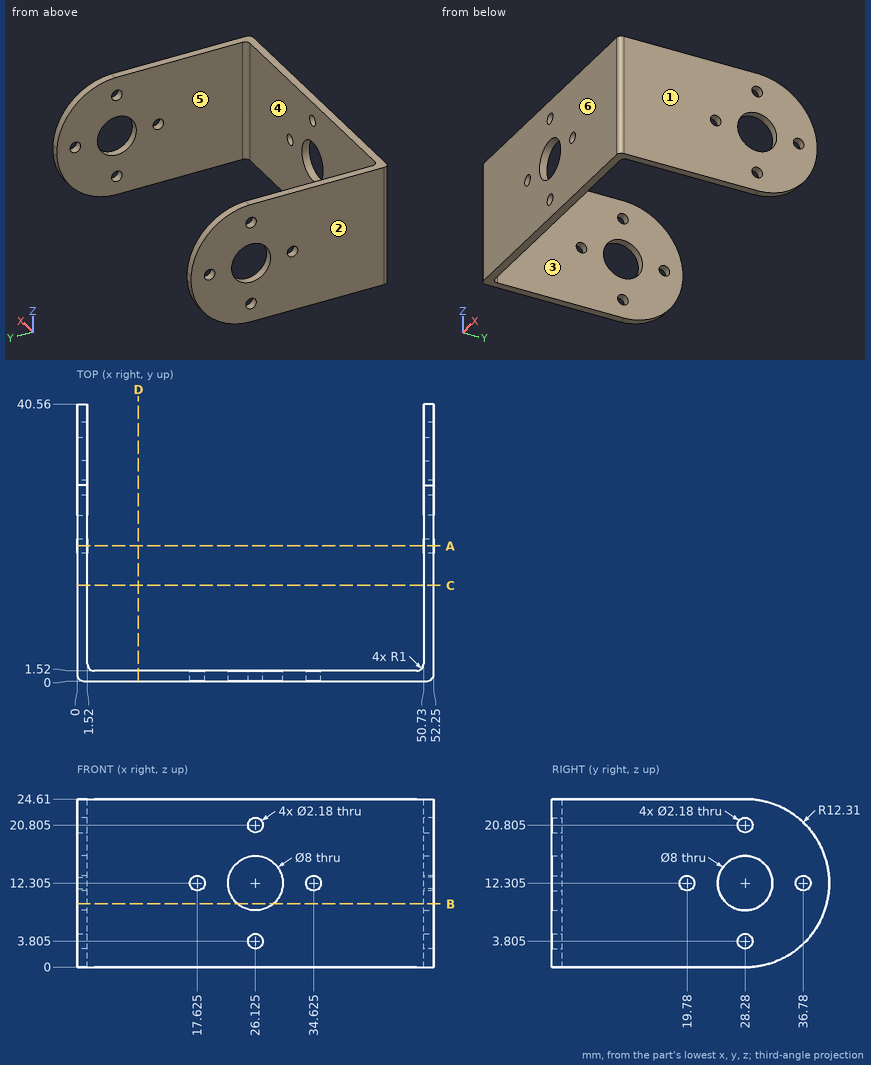
Geometry: see drawing. Coordinates: mm, zero at the bounding-box minimum. A direction names the side the tool comes from. Coordinates: 2 decimals unless noted, no trailing zeros. Write each loop counter-clockwise with the first axis right and the second up, starting at its lowest first coordinate (ties: lowest second). Pieces come first, ordered by that corner, then holes. Notation, with made-up numbers: M -32.75,53.5 L -1.75,53.5 A9 cw -1.75,64.5 Z; hole C 48.5,11 d8. An arc over 180 degrees is marked long. Use CSV: the item, a comma, the result in double quotes. Start each with the question number.
1. Mould query, pull axis X, two halves, no side actions, for the marked faces 1, 2, 3 and 4. Classes: pulls with the +X half, pulls with the -X half, needs draft (parallel to the pull), parting line crosses it, or undercut.
2. Cut plane A-A on y = 19.78. Return the cut outline in (x, z) (3 decimals), plus the area to 3 significant figures.
3. First-contact query: P1, Ø4, axis at x = 39, z = 6.5, coming from the +Y side; P2, Ø1.7, axis at y = 28.28, z = 3.805, coming from the +X side; P3, Ø12, axis at x = 46, y = 34.5, coming from the -Z side. Flat tips, straight axial feed; report the tip coordinate or a pass-through.
4. Cut plane D-D on x = 9. Return the cut outline in (y, z).
5. Cut plane B-B on z = 9.25. Return the cut outline in (x, y), plus the area to 3 significant figures.
6. Reachability of the marked faces 5 and 6 from +Z, -Z, +X, -X, +Y, -Y: full face, straight path, thin tool, end or side. Return the list, or none.
7. Ray query, probe 1 along X at (y, z) = (35.5, 14); probe 2 along Y at (x, z) = (37, 4.75); probe 3 along Z at (x, y) = (51.45, 19.78) (3 decimals). Return the intervals inside material, ascending.
8. Cut plane C-C on y = 14. Return the cut outline in (x, z).
Entries:
1,face 1,"pulls with the +X half"
1,face 2,"pulls with the -X half"
1,face 3,"undercut"
1,face 4,"undercut"
2,outline,"M 0,0 L 1.52,0 L 1.52,11.215 L 0,11.215 Z; M 0,13.395 L 1.52,13.395 L 1.52,24.61 L 0,24.61 Z; M 50.73,0 L 52.25,0 L 52.25,11.215 L 50.73,11.215 Z; M 50.73,13.395 L 52.25,13.395 L 52.25,24.61 L 50.73,24.61 Z"
2,area,"68.2 mm²"
3,P1,"y = 1.52"
3,P2,"through"
3,P3,"z = 0.26"
4,outline,"M 0,0 L 1.52,0 L 1.52,24.61 L 0,24.61 Z"
5,outline,"M 0,1 A1 ccw 1,0 L 23.54,0 L 23.54,1.52 L 2.52,1.52 A1 cw 1.52,2.52 L 1.52,25.7 L 0,25.7 Z; M 0,30.86 L 1.52,30.86 L 1.52,40.2 L 0,40.2 Z; M 28.71,0 L 51.25,0 A1 ccw 52.25,1 L 52.25,25.7 L 50.73,25.7 L 50.73,2.52 A1 cw 49.73,1.52 L 28.71,1.52 Z; M 50.73,30.86 L 52.25,30.86 L 52.25,40.2 L 50.73,40.2 Z"
5,area,"173 mm²"
6,face 5,"+Z, -Z, +Y"
6,face 6,"+Z, -Z, +X, -X, -Y"
7,probe 1,"0 to 1.52, 50.73 to 52.25"
7,probe 2,"0 to 1.52"
7,probe 3,"0 to 11.215, 13.395 to 24.61"
8,outline,"M 0,0 L 1.52,0 L 1.52,24.61 L 0,24.61 Z; M 50.73,0 L 52.25,0 L 52.25,24.61 L 50.73,24.61 Z"
